Build history of the part. All positions in model axes, mm. A direction names the side the tool comes from. Give positions to 0.01 mm unless a question says otherwise; leave off trailing zeros. Order: outer loops, then holes, each group sorted by start corner. A loop starts at its lowest first (then second) coordinate and runs counter-clockwise, first axis right, second up. Notation, with made-up numbers: (70.25, -30) -> (76.25, -30) arc R23 cw to (76.25, 3) -> close; hole circle Ø7 at (-8, 17.5). An arc over 180 degrees is marked (long way). One line per item, written item: value. Start each with the question number.
(1) Saw through at A-A on z = 1.7. Give the cut face in (x, y), plus the area to 3 significant figures.
(2) Which spindle directions (+Z, -Z, +X, -X, +Y, -Y) get a long thin tool onto all of the face, cutting with end or side? Do faces 1 (the flat face through (131, 6, 1)), 2 (the flat face through (131, 6, 0)). Say none if no direction does.
(3) Saw through at C-C on y = 6. Give the cut face in (x, z).
(4) Saw through at B-B on x = 92. Give the cut face in (y, z).
(5) Pin check, flat tip, straight feed: pin 1 (3 mm diameter, centred on x = 84.5, y = 4, fed in from +Z). Stop position of the tip, or through.
(6) Probe line 1 (Y direction, x = 131, z = 1.5); line 2 (Z direction, x = 68, y = 4.5). List the from-to ranges inside material, lowest first.
```python
from build123d import *

# Parameters (mm, degrees)
RECTANGLE008_W   = 265
RECTANGLE008_H   = 1
EXTRUDE011_DEPTH = 1
RECTANGLE007_W   = 265
RECTANGLE007_H   = 1
EXTRUDE012_DEPTH = 1
RECTANGLE009_W   = 265
RECTANGLE009_H   = 12
EXTRUDE010_DEPTH = 1


with BuildPart() as h_bottom_lip:
    # Rectangle008 → Extrude011 (new body)
    with BuildSketch(Plane.XY.offset(1)):
        with Locations((132.5, 0.5)):
            Rectangle(RECTANGLE008_W, RECTANGLE008_H)
    extrude(amount=EXTRUDE011_DEPTH)


with BuildPart() as h_top_lip:
    # Rectangle007 → Extrude012 (new body)
    with BuildSketch(Plane(origin=(0, 11, 1), x_dir=(1, 0, 0), z_dir=(0, 0, 1))):
        with Locations((132.5, 0.5)):
            Rectangle(RECTANGLE007_W, RECTANGLE007_H)
    extrude(amount=EXTRUDE012_DEPTH)


with BuildPart() as h_holder:
    # Rectangle009 → Extrude010 (new body)
    with BuildSketch(Plane.XY):
        with Locations((132.5, 6)):
            Rectangle(RECTANGLE009_W, RECTANGLE009_H)
    extrude(amount=EXTRUDE010_DEPTH)

    # Fusion005: union h_bottom_lip, h_top_lip
    add(h_bottom_lip.part)
    add(h_top_lip.part)


solid = h_holder.part
```
Results below:
1. outline: (0, 0) -> (265, 0) -> (265, 1) -> (0, 1) -> close; (0, 11) -> (265, 11) -> (265, 12) -> (0, 12) -> close
1. area: 530 mm²
2. face 1: +Z, +X, -X
2. face 2: -Z, +X, -X, +Y, -Y
3. outline: (0, 0) -> (265, 0) -> (265, 1) -> (0, 1) -> close
4. outline: (0, 0) -> (12, 0) -> (12, 2) -> (11, 2) -> (11, 1) -> (1, 1) -> (1, 2) -> (0, 2) -> close
5. pin 1: stops at z = 1
6. line 1: y = 0 to 1, 11 to 12
6. line 2: z = 0 to 1
